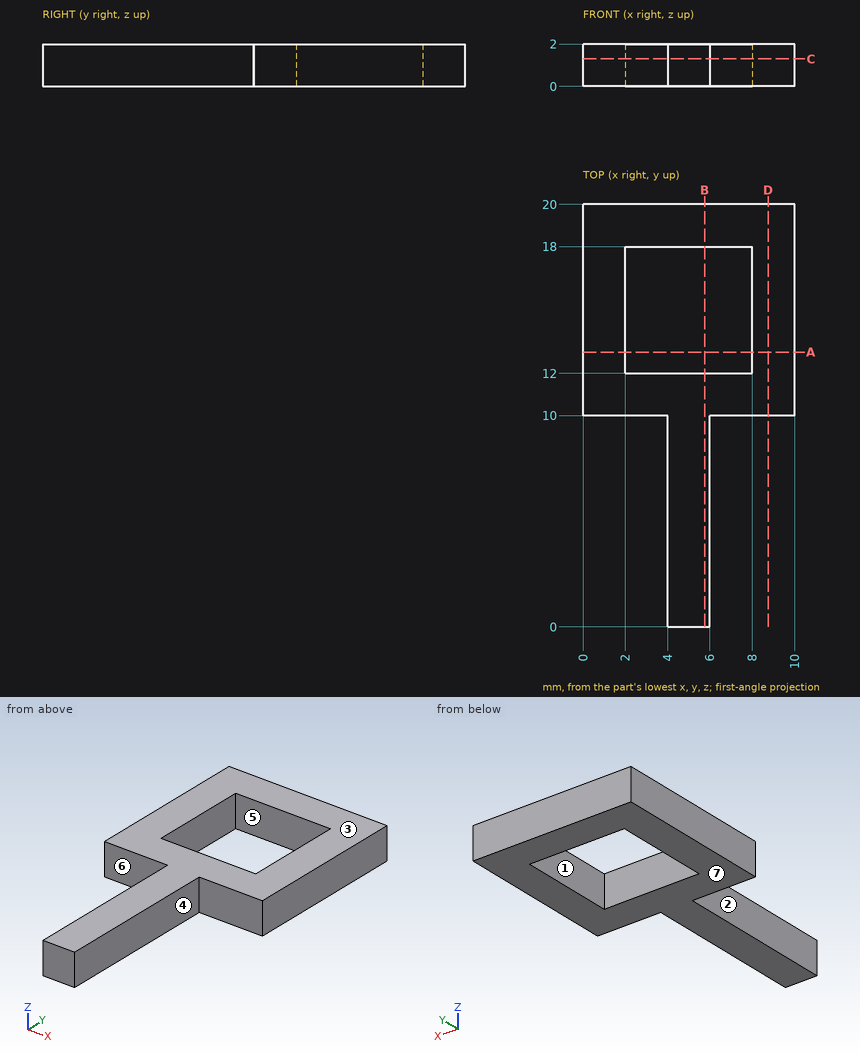
Design review of the part shown in the three views and the two pictorial views. Dimensions are in mm from the part's minimum x, y and z. A direction names the side the tool comes from. Round coordinates to 2 decimals unless told otherwise and drop trailing zeros. Order: outer loops, then holes, each group sorted by start corner. A loop starts at its lowest first (then second) coordinate and runs counter-clockwise, first axis right, second up.
Q1. Machinability: for the marked faces 1, 2, 3 and 4, which of the approach directions +Z, -Z, +X, -X, +Y, -Y give a long, thin tool a straight path to every point of the face, cutting with its end or side? Answer none if there is none.
Findings below:
face 1: +Z, -Z
face 2: +Z, -Z, -X, -Y
face 3: +Z, +X, -X, +Y, -Y
face 4: +Z, -Z, +X, -Y
Q2. We need section A-A, the plane y = 13. Give the boundary of the cut face in (x, z), plus the area to 3 significant figures.
Findings below:
outline: (0, 0) - (2, 0) - (2, 2) - (0, 2) - close; (8, 0) - (10, 0) - (10, 2) - (8, 2) - close
area: 8.00 mm2
Q3. We need section C-C, the plane z = 1.3. Give the boundary of the cut face in (x, y), plus the area to 3 significant figures.
Findings below:
outline: (0, 10) - (4, 10) - (4, 0) - (6, 0) - (6, 10) - (10, 10) - (10, 20) - (0, 20) - close; hole (2, 12) - (8, 12) - (8, 18) - (2, 18) - close
area: 84.0 mm2
Q4. Wall thickness on line 1 (Y direction, x = 3.5, z = 1.15); line 2 (X direction, y = 16.5, z = 0.95); line 3 (Y direction, x = 5.5, z = 1.35): over which ranges is each line inside the solid? List them lowest first.
Findings below:
line 1: y = 10 to 12, 18 to 20
line 2: x = 0 to 2, 8 to 10
line 3: y = 0 to 12, 18 to 20
Q5. Mouldability with a two-part tool opening along Y and no side actions: class the marked faces 5, 6 and 7 as pulls with the +Y half, pulls with the -Y half, needs draft (parallel to the pull), parting line crosses it, or undercut.
Findings below:
face 5: undercut
face 6: pulls with the -Y half
face 7: needs draft
Q6. We need section B-B, the plane x = 5.75. Give the boundary of the cut face in (y, z).
Findings below:
outline: (0, 0) - (12, 0) - (12, 2) - (0, 2) - close; (18, 0) - (20, 0) - (20, 2) - (18, 2) - close
Q7. We need section D-D, the plane x = 8.75. Give the boundary of the cut face in (y, z), plus the area to 3 significant figures.
Findings below:
outline: (10, 0) - (20, 0) - (20, 2) - (10, 2) - close
area: 20.0 mm2
Q8. Insertion check: P1, Ø0.6, axis at y = 6.5, z = 0.5, coming from the +X side; P2, Ø1, axis at y = 15, z = 0.5, coming from the -X side; P3, Ø1.5, axis at x = 7, y = 3, coming from the +Z side. Each pin has a flat end and moves straight along its axis. Give the tip position at first contact, or say it passes through.
Findings below:
P1: stops at x = 6
P2: stops at x = 0
P3: passes through
